Part print with two shaded views. Sizes in mm from the minimum x, y, z corner. Round coordinates to 2 decimals unless told otherwise and drop trailing zeros. Order: outer loops, then holes, each group sorted by start corner. A loop starts at its lowest first (then second) coordinate and runs counter-clockwise, first axis right, second up. Notation, with made-up numbers: (20.5, 19.25) -> (71.5, 19.25) arc R24 cw to (71.5, 40.25) -> close; hole circle Ø7 at (-3, -31). An arc over 180 degrees is marked (long way). Answer as a JSON object with one key per item and string values.
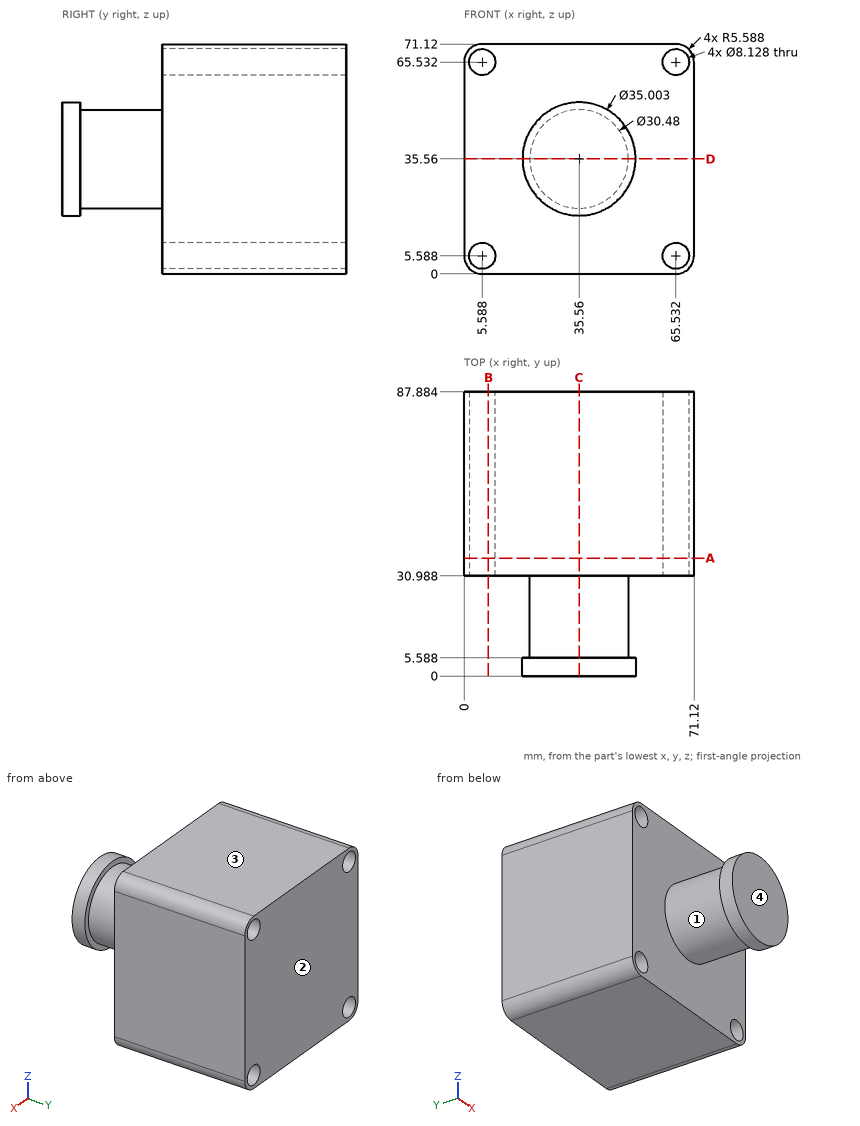
1) Probe L1, parallel to X at y = 40, z = 65.5; L2, parallel to X at y = 77, z = 64.5; L3, parallel to Y at x = 49.5, z = 46.5. List the from-to ranges inside material, lowest first. Write a range as from..to.
Checked values:
{"L1": "x = 0..1.52, 9.65..61.47, 69.6..71.12", "L2": "x = 0..1.66, 9.52..61.6, 69.46..71.12", "L3": "y = 30.99..87.88"}
2) Cut at A-A, the plane y = 36.5. Give the cut face in (x, z), plus the area to 3 significant figures.
Checked values:
{"outline": "(0, 5.59) arc R5.59 ccw to (5.59, 0) -> (65.53, 0) arc R5.59 ccw to (71.12, 5.59) -> (71.12, 65.53) arc R5.59 ccw to (65.53, 71.12) -> (5.59, 71.12) arc R5.59 ccw to (0, 65.53) -> close; hole circle Ø8.13 at (5.59, 5.59); hole circle Ø8.13 at (5.59, 65.53); hole circle Ø8.13 at (65.53, 5.59); hole circle Ø8.13 at (65.53, 65.53)", "area": "4,820 mm²"}
3) Cut at C-C, the plane x = 35.56. Give the cut face in (y, z).
Checked values:
{"outline": "(0, 18.06) -> (5.59, 18.06) -> (5.59, 20.32) -> (30.99, 20.32) -> (30.99, 0) -> (87.88, 0) -> (87.88, 71.12) -> (30.99, 71.12) -> (30.99, 50.8) -> (5.59, 50.8) -> (5.59, 53.06) -> (0, 53.06) -> close"}
4) Pull direction Y, two halves, no side cores. Call the marked faces 1, 2, 3 and 4: pulls with the +Y half, pulls with the -Y half, needs draft (parallel to the pull), parting line crosses it, or undercut.
Checked values:
{"face 1": "undercut", "face 2": "pulls with the +Y half", "face 3": "needs draft", "face 4": "pulls with the -Y half"}
5) Cut at D-D, the plane z = 35.56. Give the cut face in (x, y).
Checked values:
{"outline": "(0, 30.99) -> (20.32, 30.99) -> (20.32, 5.59) -> (18.06, 5.59) -> (18.06, 0) -> (53.06, 0) -> (53.06, 5.59) -> (50.8, 5.59) -> (50.8, 30.99) -> (71.12, 30.99) -> (71.12, 87.88) -> (0, 87.88) -> close"}
6) Cut at B-B, the plane x = 7.5. Give the cut face in (y, z), plus the area to 3 significant figures.
Checked values:
{"outline": "(30.99, 0) -> (87.88, 0) -> (87.88, 2) -> (30.99, 2) -> close; (30.99, 9.17) -> (87.88, 9.17) -> (87.88, 61.95) -> (30.99, 61.95) -> close; (30.99, 69.12) -> (87.88, 69.12) -> (87.88, 71.12) -> (30.99, 71.12) -> close", "area": "3,230 mm²"}
7) Flat gauge pins, fed straight in: pin 1 Ø6 at (x, z) = (57, 54.5) entering from -Y; pin 2 Ø5 at (x, z) = (65.532, 65.532) entering from -Y. Where does each tip first touch, or does it go through?
Checked values:
{"pin 1": "stops at y = 30.99", "pin 2": "passes through"}
